```python
from build123d import *

# Parameters (mm, degrees)
F1_DEPTH = 77.724


with BuildPart() as f1:
    # F0 (on Right) → F1 (new body, symmetric)
    with BuildSketch(Plane.YZ):
        Polygon((-6.2865, -39.878), (6.2865, -39.878), (6.2865, -23.622), (21.0566, -23.622), (21.0566, 36.83), (21.0566, 39.878), (9.2964, 36.83), (-34.8996, 36.83), (-21.0566, 27.686), (-21.0566, -23.622), (-6.2865, -23.622), align=None)
    extrude(amount=F1_DEPTH, both=True)


solid = f1.part
```
Could you check a few things on this model? Use its own coordinates, in mm. A direction names the side the tool comes from. Coordinates: 2 decimals unless noted, no trailing zeros. Order: outer loops, then holes, each group sorted by start corner. A loop starts at its lowest first (then second) coordinate and runs counter-clockwise, first axis right, second up. Notation, with made-up numbers: M 54,56.25 L 64,56.25 A32 ccw 64,86.25 Z; hole C -16.5,59 d9. An arc over 180 degrees is marked long. Use a Markdown table: item, result. Add a question column.
Q1. I want a section at B-B on z = -31.5. List the corners of the cut face in (x, y) for me, then the cut area to 3 significant figures.
Q2. If I drill on L1, parallel to Z at x = 64.5, y = 1.5; L2, parallel to Z at x = -43.5, y = -15.5; L3, parallel to Y at x = -40.5, z = 1, over which ranges is the centre line in solid material (lowest first)?
Q3. I want a section at C-C on y = -17. List the corners of the cut face in (x, z) for me.
Q4. I'm going to push flat-ended pins straight in: pin 1 (18 mm diameter, centred on x = -22.5, z = -28, fed in from -Y); pin 2 (16 mm diameter, centred on x = -20, y = -13, fed in from -Z); pin 3 (13 mm diameter, centred on x = 4, z = -32.5, fed in from +Y); pin 4 (12 mm diameter, centred on x = 37, y = 15.5, fed in from -Z). Where does each tip first touch, or does it pass through?
Q5. I want a section at A-A on x = 1.5. List the corners of the cut face in (y, z) for me, then the cut area to 3 significant figures.
Q6. Which directions (+Z, -Z, +X, -X, +Y, -Y) give clear straight access to the entire face, cutting with the end or side of a thin tool? Please do faces 1 (the flat face through (1, 6.286, -32)), 2 (the flat face through (1, -14, -23.622)), 3 (the flat face through (1, -12, 36.83)).
Checked values:
| question | item | result |
|---|---|---|
| 1 | outline | M -77.72,-6.29 L 77.72,-6.29 L 77.72,6.29 L -77.72,6.29 Z |
| 1 | area | 1,950 mm² |
| 2 | L1 | -39.88 to 36.83 |
| 2 | L2 | -23.62 to 36.83 |
| 2 | L3 | -21.06 to 21.06 |
| 3 | outline | M -77.72,-23.62 L 77.72,-23.62 L 77.72,36.83 L -77.72,36.83 Z |
| 4 | pin 1 | y = -21.06 |
| 4 | pin 2 | z = -39.88 |
| 4 | pin 3 | y = 6.29 |
| 4 | pin 4 | z = -23.62 |
| 5 | outline | M -34.9,36.83 L -21.06,27.69 L -21.06,-23.62 L -6.29,-23.62 L -6.29,-39.88 L 6.29,-39.88 L 6.29,-23.62 L 21.06,-23.62 L 21.06,39.88 L 9.3,36.83 Z |
| 5 | area | 2,830 mm² |
| 6 | face 1 | -Z, +X, -X, +Y |
| 6 | face 2 | -Z, +X, -X, -Y |
| 6 | face 3 | +Z, +X, -X, -Y |
